Part model, mm, in its own coordinate system. Face numbers are marked on the shaded views. A direction names the side the tool comes from. Round coordinates to 2 decimals unless told otherwise and drop trailing zeros. Loops run counter-clockwise (first coordinate to the right, second up) from the corner with the lowest first, then second, coordinate; pieces in that order, holes last.
1) Band-saw the part on D-D, the plane y = 3.5. Write the cut outline in (x, z), then the cut area to 3 significant figures.
2) Probe line 1 (Z direction, x = 2.75, y = 6); line 2 (X direction, y = 5.75, z = 14.5); line 3 (X direction, y = 10.75, z = 16). List the from-to ranges inside material, lowest first.
3) Drop flat-ended pins along their axis: P1, Ø1.8, axis at x = -1, z = -4, coming from the +Y side; P2, Ø2.5, axis at x = -6.5, z = -23, coming from the +Y side; P3, Ø0.8, axis at x = 0.5, y = 10.5, coming from the +Z side; P4, Ø1.5, axis at y = 6.5, z = -8, coming from the -X side. Give the stop position or say it passes through.
4) 3-axis set-ups, long thin cutter, end or side, ignore diameter. For the marked faces 1, 2, 3, 4 and 5: which of +Z, -Z, +X, -X, +Y, -Y reach the whole face in a straight line?
5) Band-saw the part on A-A, the plane y = 7. Write the cut outline in (x, z), then the cut area to 3 significant figures.
6) Mould opens along Z. For the marked faces 6, 7 and 8 say: +Z half, -Z half, draft (parallel to the pull), parting line (faces both ways), or undercut.
7) Band-saw the part on B-B, the plane x = -1. Write the cut outline in (y, z).
8) Band-saw the part on C-C, the plane z = 9. Write the cut outline in (x, y).
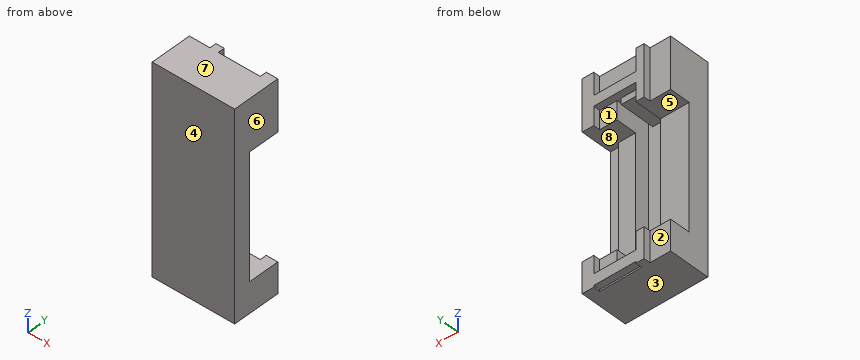
Autodesk Fusion 360 part; units mm, degrees
sketch "Sketch1" plane through (0, 0, 0) normal (0, 1, 0) x (1, 0, 0)
  line L0 (10, -25) -> (-10, -25)
  line L1 (-10, -25) -> (-10, 25)
  line L2 (-10, 25) -> (10, 25)
  line L3 (10, 25) -> (10, -25)
  line L4 (10, -25) -> (-10, 25) construction
  line L5 (-10, -25) -> (10, 25) construction
  line L6 (0, 25) -> (0, -25) construction
  line L7 (-3, 25) -> (-3, -25)
  line L8 (3, 25) -> (3, -25)
  line L9 (7.2, 25) -> (7.2, -25)
  line L10 (-5, 25) -> (-5, -25)
  line L11 (-10, -12.6) -> (10, -12.6)
  line L12 (-10, 17.6) -> (10, 17.6)
  line L13 (10, 24.6) -> (-10, 24.6)
  line L14 (10, -19.6) -> (-10, -19.6)
  line L15 (-5, 21.9) -> (8.76, 21.9)
  line L16 (-10, 0) -> (10, 0) construction
  line L17 (-5, -17.1) -> (7.2, -17.1)
  line L18 (-3, 20.4) -> (2, 20.4)
  line L19 (2, 20.4) -> (2, 21.9)
  line L20 (2, 21.9) -> (-3, 21.9)
  line L21 (-3, 21.9) -> (-3, 20.4)
  line L22 (-3, -17.1) -> (2, -17.1)
  line L23 (2, -17.1) -> (2, -15.6)
  line L24 (2, -15.6) -> (-3, -15.6)
  line L25 (-3, -15.6) -> (-3, -17.1)
  line L26 (8.4, 17.6) -> (8.4, -12.6)
  dimension "d1" = 50
  dimension "d2" = 20
  dimension "d3" = 3
  dimension "d8" = 2.8
  dimension "d9" = 2
  dimension "d16" = 12.4
  dimension "d17" = 7.4
  dimension "d30" = 7
  dimension "d31" = 7
  dimension "d35" = 2.7
  dimension "d36" = 2.5
  dimension "d46" = 1.5
  dimension "d47" = 5
  dimension "d48" = 1.5
  dimension "d49" = 5
  dimension "d53" = 1.2
extrude "Extrude1" add sketch "Sketch1" along normal blind 1.5
extrude "Extrude2" add sketch "Sketch1" along normal blind 10 contours L0 L3 L9 L14 | L0 L8 L9 L14 | L3 L9 L11 L14 | L8 L9 L14 L17 | L3 L11 L12 L26 | L0 L7 L10 L14 | L8 L9 L11 L17 | L3 L9 L12 L13 | L9 L11 L12 L26 | L0 L1 L10 L14 | L7 L10 L14 L17 | L8 L9 L11 L12 | L2 L3 L9 L13 | L1 L10 L11 L14 | L7 L10 L11 L17 L25 | L8 L9 L12 L15 | L2 L8 L9 L13 | L8 L9 L13 L15 | L7 L10 L11 L12 | L1 L10 L11 L12 | L7 L10 L12 L15 L21 | L2 L7 L10 L13 | L7 L10 L13 L15 | L1 L10 L12 L13 | L1 L2 L10 L13
extrude "Extrude3" add sketch "Sketch1" along normal blind 1.6 from surface at 10 contours L0 L3 L9 L14 | L3 L9 L11 L14 | L3 L11 L12 L26 | L3 L9 L12 L13 | L9 L11 L12 L26 | L2 L3 L9 L13
extrude "Extrude4" add sketch "Sketch1" along normal blind 1.6 from surface at 10 contours L0 L7 L10 L14 | L7 L10 L14 L17 | L7 L10 L11 L17 L25 | L7 L10 L11 L12 | L7 L10 L12 L15 L21 | L2 L7 L10 L13 | L7 L10 L13 L15
extrude "Extrude6" cut sketch "Sketch1" against normal blind 5 from surface at 11.6 contours L3 L11 L12 L26 | L9 L11 L12 L26 | L7 L10 L11 L12
extrude "Extrude7" cut sketch "Sketch1" against normal blind 5 from surface at 10 contours L3 L11 L12 L26 | L9 L11 L12 L26 | L7 L10 L11 L12 | L1 L10 L11 L12
extrude "Extrude8" cut sketch "Sketch1" against normal blind 5 from surface at 10 contours L3 L11 L12 L26 | L9 L11 L12 L26 | L8 L9 L11 L12
extrude "Extrude9" add sketch "Sketch1" along normal up to surface (8.5 mm away) from surface at 1.5 contours L0 L7 L8 L14 | L2 L7 L8 L13
extrude "Extrude10" add sketch "Sketch1" along normal up to surface (8.5 mm away) from surface at 1.5 contours L7 L8 L14 L17 L22 | L7 L8 L13 L15 L20
extrude "Extrude11" add sketch "Sketch1" along normal up to surface (1.6 mm away) from surface at 10 contours L8 L9 L13 L15 | L7 L8 L13 L15 L20 | L7 L10 L13 L15
extrude "Extrude12" add sketch "Sketch1" along normal up to surface (1.6 mm away) from surface at 10 contours L8 L9 L14 L17 | L7 L8 L14 L17 L22
extrude "Extrude13" add sketch "Sketch1" along normal up to surface (8.5 mm away) from surface at 1.5 contours L7 L17 L22 L23 L24 L25 | L7 L15 L18 L19 L20 L21
extrude "Extrude14" cut sketch "Sketch1" against normal blind 1 from surface at 5 contours L3 L11 L12 L26 | L9 L11 L12 L26
Reported:
1. outline: (-10, -25) - (10, -25) - (10, 25) - (-10, 25) - close; hole (-3, -20.4) - (2, -20.4) - (2, -21.9) - (3, -21.9) - (3, 17.1) - (2, 17.1) - (2, 15.6) - (-3, 15.6) - close
1. area: 781 mm2
2. line 1: z = -25 to -21.9, 17.1 to 25
2. line 2: x = -10 to -3, 3 to 10
2. line 3: x = -5 to -3, 7.2 to 10
3. P1: stops at y = 1.5
3. P2: stops at y = 10
3. P3: stops at z = 19.6
3. P4: passes through
4. face 1: +Y
4. face 2: +Z, -Z, -X, +Y
4. face 3: -Z, +X, -X, +Y, -Y
4. face 4: +Z, -Z, +X, -X, -Y
4. face 5: +X, -X, +Y
5. outline: (-10, -25) - (10, -25) - (10, -17.6) - (3, -17.6) - (3, -21.9) - (2, -21.9) - (2, -20.4) - (-3, -20.4) - (-3, -17.6) - (-10, -17.6) - close; (-10, 12.6) - (-3, 12.6) - (-3, 15.6) - (2, 15.6) - (2, 17.1) - (3, 17.1) - (3, 12.6) - (10, 12.6) - (10, 25) - (-10, 25) - close
5. area: 358 mm2
6. face 6: draft
6. face 7: +Z half
6. face 8: undercut
7. outline: (0, -25) - (10, -25) - (10, -24.6) - (11.6, -24.6) - (11.6, -21.9) - (10, -21.9) - (10, -20.4) - (1.5, -20.4) - (1.5, 15.6) - (10, 15.6) - (10, 17.1) - (11.6, 17.1) - (11.6, 19.6) - (10, 19.6) - (10, 25) - (0, 25) - close
8. outline: (-10, 0) - (10, 0) - (10, 4) - (7.2, 4) - (7.2, 5) - (3, 5) - (3, 1.5) - (-3, 1.5) - (-3, 5) - (-10, 5) - close
